The model under review builds one solid part; all positions refer to its coordinate system, in mm. A direction names the side the tool comes from. Round coordinates to 2 decimals unless told otherwise and drop trailing zeros. Write each loop counter-clockwise with the first axis right and the second up, starting at its lowest first coordinate (ties: lowest second). Pieces come first, ordered by that corner, then holes. Notation, with made-up numbers: (55.25, -18) - (85.25, -18) arc R24 ccw to (85.25, 4) - close; hole circle Ø11 at (55.25, -21.75). An arc over 180 degrees is marked (long way). Write each question's results on one line, items separated by ' | '.
```python
from build123d import *

# Parameters (mm, degrees)
SKETCH1_W           = 60
SKETCH1_H           = 20
BOSS_EXTRUDE5_DEPTH = 10
SKETCH4_W           = 10
SKETCH4_H           = 20
BOSS_EXTRUDE6_DEPTH = 10
SKETCH5_W           = 10
SKETCH5_H           = 10
CUT_EXTRUDE4_DEPTH  = 3
SKETCH6_R           = 2
CUT_EXTRUDE5_DEPTH  = 14
FILLET2_R           = 3


with BuildPart() as part:
    # Sketch1 → Boss-Extrude5 (new body)
    with BuildSketch(Plane.XY):
        Rectangle(SKETCH1_W, SKETCH1_H)
        Polygon((-23.181980124, 7.42462107), (-27.42462133, 3.181980902), (-24.242640893, 3.09e-07), (-27.424621334, -3.181979354), (-23.181981665, -7.424621059), (-20.00000031, -4.242640483), (-16.818019873, -7.424621076), (-12.575378663, -3.181980905), (-15.757358789, 0), (-12.575378649, 3.181979361), (-16.818018342, 7.424621043), (-19.999999246, 4.242640917), align=None, mode=Mode.SUBTRACT)
        Polygon((23, 7.5), (17, 7.5), (17, 3), (12.5, 3), (12.5, -3), (17, -3), (17, -7.5), (23, -7.5), (23, -3), (27.5, -3), (27.5, 3), (23, 3), align=None, mode=Mode.SUBTRACT)
    extrude(amount=BOSS_EXTRUDE5_DEPTH)

    # Sketch4 → Boss-Extrude6 (add)
    with BuildSketch(Plane(origin=(30, 0, 0), x_dir=(0, 0, -1), z_dir=(1, 0, 0))):
        with Locations((-5, 0)):
            Rectangle(SKETCH4_W, SKETCH4_H)
    extrude(amount=BOSS_EXTRUDE6_DEPTH)

    # Sketch5 → Cut-Extrude4 (cut)
    with BuildSketch(Plane(origin=(40, 0, 0), x_dir=(0, 0, -1), z_dir=(1, 0, 0))):
        with Locations((-5, 0)):
            Rectangle(SKETCH5_W, SKETCH5_H)
    extrude(amount=-CUT_EXTRUDE4_DEPTH, mode=Mode.SUBTRACT)

    # Sketch6 → Cut-Extrude5 (cut)
    with BuildSketch(Plane(origin=(37, 0, 0), x_dir=(0, 0, -1), z_dir=(1, 0, 0))):
        with Locations((-5, 0)):
            Circle(SKETCH6_R)
    extrude(amount=-CUT_EXTRUDE5_DEPTH, mode=Mode.SUBTRACT)

    # Fillet2
    fillet2_edges = [part.edges().sort_by_distance(p)[0] for p in [
        (-30, 10, 5),
        (-30, -10, 5),
        (40, 10, 5),
        (40, -10, 5),
    ]]
    fillet(fillet2_edges, radius=FILLET2_R)


solid = part.part
```
Q1. The part is to be moulded in two halves that separate along X. For faces 4 (the cylindrical face through (32.3, -1.2, 6.6)), 5 (the cylindrical face through (-29.1, -9.14, 5.07)), 6 (the flat face through (-18.43, -5.81, 4.93)), say which applies: released by +X, released by -X, zero draft, split by the parting line, or undercut.
Evaluation:
face 4: zero draft | face 5: released by -X | face 6: undercut
Q2. We need section B-B (y = 1). State the section outline as (x, z) points.
Evaluation:
outline: (-30, 0) - (-25.24, 0) - (-25.24, 10) - (-30, 10) - close; (-14.76, 0) - (12.5, 0) - (12.5, 10) - (-14.76, 10) - close; (27.5, 0) - (37, 0) - (37, 3.27) - (27.5, 3.27) - close; (27.5, 6.73) - (37, 6.73) - (37, 10) - (27.5, 10) - close
Q3. Insertion check: P1, Ø3, axis at y = 1.5, z = 5.5, coming from the +X side; P2, Ø2.5, axis at x = 39, z = 4.5, coming from the -Y side. Each pin has a flat end and moves straight along its axis. Give the tip position at first contact, or say it passes through.
Evaluation:
P1: stops at x = 37 | P2: stops at y = -9.9
Q4. We need section C-C (z = 1.25). State how many separate pieces and enclosed holes the cut face has, plus the area to 3 significant figures.
Evaluation:
separate pieces: 1 | enclosed holes: 2 | area: 1,070 mm^2
Q5. Tool access review of faces 1 (the flat face through (12.5, 0, 5)), 2 (the flat face through (39, -5, 5)), 3 (the flat face through (-30, 0, 5)): name each direction out of +Z, -Z, +X, -X, +Y, -Y from which nothing blocks a thin tool from reaching the whole face with its end or side.
Evaluation:
face 1: +Z, -Z | face 2: +Z, -Z, +X | face 3: +Z, -Z, -X, +Y, -Y
Q6. We need section A-A (x = 26.5). State the section outline as (y, z) points.
Evaluation:
outline: (-10, 0) - (-3, 0) - (-3, 10) - (-10, 10) - close; (3, 0) - (10, 0) - (10, 10) - (3, 10) - close
Q7. We need section D-D (x = 19.5). State the section outline as (y, z) points.
Evaluation:
outline: (-10, 0) - (-7.5, 0) - (-7.5, 10) - (-10, 10) - close; (7.5, 0) - (10, 0) - (10, 10) - (7.5, 10) - close
Q8. For probe 1 along Y at (x, z) = (32.75, 5); probe 2 along X at (y, z) = (-1.25, 8.5); probe 3 along Y at (x, z) = (14, 5), list the stretches that pass through material, from the lowest coordinate up.
Evaluation:
probe 1: y = -10 to -2, 2 to 10 | probe 2: x = -30 to -25.49, -14.51 to 12.5, 27.5 to 37 | probe 3: y = -10 to -3, 3 to 10
